The listing builds one solid part. Answer for the finished solid, in the listing's coordinates (mm). A direction names the side the tool comes from. Round coordinates to 2 decimals unless told otherwise and drop trailing zeros. Write each loop counter-clockwise with the first axis right and the second up, starting at its lowest first coordinate (ties: lowest second). Pieces come first, ordered by that corner, then holes. Notation, with made-up numbers: M 67,4 L 104,4 A14 cw 104,31 Z; hole C -5.75,48.5 d10. An arc over 180 degrees is marked long. Write each question's results on one line, items separated by ' | '.
from build123d import *

# Parameters (mm, degrees)
SKETCH_W     = 49.4
SKETCH_H     = 52
SKETCH_R     = 13
PAD_DEPTH    = 3
SKETCH001_R  = 3.1
POCKET_DEPTH = 2.4


with BuildPart() as part:
    # Sketch → Pad (new body)
    with BuildSketch(Plane.XY):
        with Locations((24.7, 26)):
            Rectangle(SKETCH_W, SKETCH_H)
        with Locations((24.7, 26)):
            Circle(SKETCH_R, mode=Mode.SUBTRACT)
    extrude(amount=PAD_DEPTH)

    # Sketch001 → Pocket (cut)
    with BuildSketch(Plane.XY):
        with Locations((24.7, 6)):
            Circle(SKETCH001_R)
        with Locations((6, 26)):
            Circle(SKETCH001_R)
        with Locations((43.4, 26)):
            Circle(SKETCH001_R)
    extrude(amount=POCKET_DEPTH, mode=Mode.SUBTRACT)


solid = part.part
1) Find the intervals of material crossed by line 1 (Y direction, x = 24.7, z = 0.75); line 2 (Y direction, x = 6, z = 1.3); line 3 (X direction, y = 24.5, z = 1.55), in increasing order.
Return value:
line 1: 0 to 2.9, 9.1 to 13, 39 to 52 | line 2: 0 to 22.9, 29.1 to 52 | line 3: 0 to 3.29, 8.71 to 11.79, 37.61 to 40.69, 46.11 to 49.4
2) Section A-A (x = 24.7) is taken. Determine the outline of the cut face in (y, z).
Return value:
outline: M 0,0 L 2.9,0 L 2.9,2.4 L 9.1,2.4 L 9.1,0 L 13,0 L 13,3 L 0,3 Z; M 39,0 L 52,0 L 52,3 L 39,3 Z
3) The mould has two halves that part along X. Classify faces 3 (the face through (37.1, 29.9, 1.5)), 4 (the face through (49.4, 26, 1)), 5 (the face through (19, 38, 3)): +X half, -X half, draft (parallel to the pull), parting line (faces both ways), or undercut.
Return value:
face 3: undercut | face 4: +X half | face 5: draft
4) Section D-D (x = 6) is taken. Determine the outline of the cut face in (y, z).
Return value:
outline: M 0,0 L 22.9,0 L 22.9,2.4 L 29.1,2.4 L 29.1,0 L 52,0 L 52,3 L 0,3 Z
5) A tool of negligible diameter and unlimited length cuts with its end or side. For faces 1 (the face through (2.9, 26.1, 1.2)), 2 (the face through (0, 26, 1)), from which of +Z, -Z, +X, -X, +Y, -Y can it reach the whole face along a straight path? Write none if from no direction.
Return value:
face 1: -Z | face 2: +Z, -Z, -X, +Y, -Y
6) Section C-C (z = 1) is taken. Determine the outline of the cut face in (x, y).
Return value:
outline: M 0,0 L 49.4,0 L 49.4,52 L 0,52 Z; hole C 6,26 d6.2; hole C 24.7,26 d26; hole C 24.7,6 d6.2; hole C 43.4,26 d6.2
7) Each of these flat-tipped pins is pushed along its axis until it touches: pin 1 (2 mm diameter, centred on x = 26, y = 42.5, fed in from -Z); pin 2 (21 mm diameter, centred on x = 24.7, y = 26, fed in from -Z); pin 3 (1.9 mm diameter, centred on x = 5.5, y = 25.5, fed in from -Z). Where does it stop, or does it pass through?
Return value:
pin 1: z = 0 | pin 2: through | pin 3: z = 2.4
8) Section B-B (y = 26) is taken. Determine the outline of the cut face in (x, z).
Return value:
outline: M 0,0 L 2.9,0 L 2.9,2.4 L 9.1,2.4 L 9.1,0 L 11.7,0 L 11.7,3 L 0,3 Z; M 37.7,0 L 40.3,0 L 40.3,2.4 L 46.5,2.4 L 46.5,0 L 49.4,0 L 49.4,3 L 37.7,3 Z
